Build history of the part. All positions in model axes, mm. Round coordinates to 2 decimals unless told otherwise and drop trailing zeros. Write each loop counter-clockwise with the first axis right and the second up, starting at its lowest first coordinate (ties: lowest second). Pieces come first, ordered by that corner, then holes.
Item 1: Band-saw the part on A-A, the plane z = -475. Write the cut outline in (x, y), then the cut area to 3 significant figures.
Item 2: Band-saw the part on B-B, the plane x = -600. Write the cut outline in (y, z).
Item 3: Band-saw the part on C-C, the plane y = 3.5. Count the separate pieces of the cut face and the enclosed holes in it, then the cut area to 3 significant figures.
Item 4: Wall check: probe 1 along Z at (x, y) = (-199.5, 3.85); probe 2 along X at (y, z) = (3.15, -649.5); probe 3 along X at (y, z) = (1.65, -334.5). Give the ranges that are in metal, low to high.
Item 5: Drop a flat-ended pin along its axis: pin 1 Ø3.5 at (x, z) = (-360, -569) entering from -Y. Give the stop position or say it passes through.
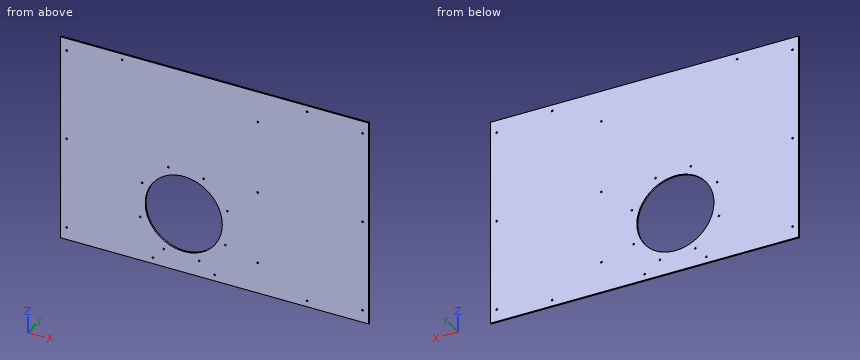
Autodesk Inventor part; units mm, degrees
ref_plane "YZ Plane" through (0, 0, 0) normal (1, 0, 0) x (0, 1, 0)
ref_plane "XZ Plane" through (0, 0, 0) normal (0, 1, 0) x (-1, 0, 0)
ref_plane "XY Plane" through (0, 0, 0) normal (0, 0, 1) x (1, 0, 0)
sketch "Sketch1" plane through (0, 0, 0) normal (0, 1, 0) x (-1, 0, 0)
  line L0 (0, 0) -> (1000, 0)
  line L1 (1000, 0) -> (1000, -669)
  line L2 (1000, -669) -> (0, -669)
  line L3 (0, -669) -> (0, 0)
  dimension "d0" = 1000
  dimension "d1" = 669
extrude "Extrusion1" add sketch "Sketch1" along normal blind 5
sketch "Sketch2" plane through (0, 5, 0) normal (0, 1, 0) x (1, 0, 0)
  circle A0 centre (-600, 475) radius 125
  line L0 (-1000, 0) -> (0, 0)
  line L1 (0, 0) -> (0, 669)
  dimension "d4" = 250
  dimension "d5" = 475
  dimension "d6" = 600
extrude "Extrusion2" cut sketch "Sketch2" against normal through all
sketch "Sketch3" plane through (0, 5, 0) normal (0, 1, 0) x (1, 0, 0)
  line L0 (0, 0) -> (0, 669)
  line L1 (-1000, 0) -> (0, 0)
  line L2 (0, 669) -> (-1000, 669)
  line L3 (-1000, 669) -> (-1000, 0)
  point P0 (-20, 40)
  point P1 (-20, 334.5)
  point P2 (-20, 629)
  point P3 (-980, 40)
  point P4 (-980, 334.5)
  point P5 (-980, 629)
  dimension "d9" = 20
  dimension "d11" = 40
  dimension "d12" = 334.5
  dimension "d13" = 20
  dimension "d14" = 40
  dimension "d15" = 20
  dimension "d16" = 40
  dimension "d17" = 20
  dimension "d18" = 334.5
  dimension "d19" = 20
  dimension "d20" = 20
  dimension "d21" = 40
hole "Hole1" at (-20, 5, -40) at (-20, 5, -334.5) at (-20, 5, -629) at (-980, 5, -40) at (-980, 5, -334.5) at (-980, 5, -629) direction (0, -1, 0) diameter 5.5 end through all
sketch "Sketch5" plane through (0, 5, 0) normal (0, 1, 0) x (1, 0, 0)
  point P0 (0, 0)
sketch "Sketch6" plane through (0, 5, 0) normal (0, 1, 0) x (1, 0, 0)
  line L0 (-1000, 0) -> (0, 0)
  line L1 (0, 0) -> (0, 669)
  circle A0 centre (-600, 475) radius 125
  point P0 (-650, 333.5786)
  dimension "d48" = 650
  dimension "d49" = 150
hole "Hole3" at (-650, 5, -333.5786) direction (0, -1, 0) diameter 5.5 end through all
pattern_circular "Circular Pattern1" count 8 over 360 about axis through (-600, 5, -475) along (0, -1, 0) of "Hole3"
sketch "Sketch7" plane through (0, 5, 0) normal (0, 1, 0) x (1, 0, 0)
  line L0 (-1000, 0) -> (0, 0)
  line L1 (0, 0) -> (0, 669)
  line L2 (0, 669) -> (-1000, 669)
  point P0 (-800, 19.5)
  point P1 (-700, 649.5)
  dimension "d54" = 19.5
  dimension "d55" = 700
  dimension "d56" = 800
  dimension "d68" = 19.5
hole "Hole4" at (-700, 5, -649.5) at (-800, 5, -19.5) direction (0, -1, 0) diameter 5.5 end through all
sketch "Sketch8" plane through (0, 5, 0) normal (0, 1, 0) x (1, 0, 0)
  line L0 (-1000, 0) -> (0, 0)
  line L1 (0, 0) -> (0, 669)
  line L2 (0, 669) -> (-1000, 669)
  point P0 (-200, 19.5)
  point P1 (-200, 649.5)
  dimension "d80" = 19.5
  dimension "d81" = 200
  dimension "d82" = 200
  dimension "d83" = 19.5
hole "Hole5" at (-200, 5, -19.5) at (-200, 5, -649.5) direction (0, -1, 0) diameter 5.5 end through all
sketch "Sketch9" plane through (0, 5, 0) normal (0, 1, 0) x (1, 0, 0)
  line L0 (0, 0) -> (0, 669)
  line L1 (0, 669) -> (-1000, 669)
  point P0 (-500, 649.5)
  dimension "d84" = 500
  dimension "d85" = 19.5
hole "Hole6" at (-500, 5, -649.5) direction (0, -1, 0) diameter 5.5 end through all
sketch "Sketch10" plane through (0, 5, 0) normal (0, 1, 0) x (1, 0, 0)
  line L0 (-1000, 0) -> (0, 0)
  line L1 (0, 669) -> (-1000, 669)
  line L2 (0, 0) -> (0, 669)
  point P0 (-360, 100)
  point P1 (-360, 569)
  point P2 (-360, 334.5)
  dimension "d93" = 100
  dimension "d94" = 334.5
  dimension "d95" = 100
  dimension "d103" = 360
  dimension "d104" = 360
  dimension "d105" = 360
hole "Hole7" at (-360, 5, -100) at (-360, 5, -334.5) at (-360, 5, -569) direction (0, -1, 0) diameter 5.5 end through all
properties part number "RearPanel"
Results:
1. outline: (-1000, 0) - (-725, 0) - (-725, 5) - (-1000, 5) - close; (-475, 0) - (0, 0) - (0, 5) - (-475, 5) - close
1. area: 3,750 mm2
2. outline: (0, -669) - (5, -669) - (5, -600) - (0, -600) - close; (0, -350) - (5, -350) - (5, 0) - (0, 0) - close
3. separate pieces: 1
3. enclosed holes: 23
3. area: 619,000 mm2
4. probe 1: z = -669 to -652.2, -646.8 to -22.2, -16.8 to 0
4. probe 2: x = -1000 to -702.75, -697.25 to -502.75, -497.25 to -202.75, -197.25 to 0
4. probe 3: x = -1000 to -982.75, -977.25 to -652.59, -647.41 to -362.75, -357.25 to -22.75, -17.25 to 0
5. pin 1: passes through
